```python
from build123d import *

# Parameters (mm, degrees)
BASES_R                     = 6.35
BASE_DEPTH                  = 5.4
TOPBORES_R                  = 1.4
TOP_BORE_DEPTH              = 11.478788098
HORN_START                  = -2.5
HORN_HALF_DEPTH             = 2.5
HORNATTACHS_R               = 0.5
HORN_ATTACH_DEPTH           = 21.913031822
HA_LP_COUNT                 = 4
HA_LP_PITCH                 = 3
HORN_BODIES_COPY_1_SKETCH_R = 0.5
HORN_BODIES_COPY_1_DEPTH    = 21.913031822
HORN_BODIES_COPY_2_SKETCH_R = 0.5
HORN_BODIES_COPY_2_DEPTH    = 21.913031822
HORN_BODIES_COPY_3_SKETCH_R = 0.5
HORN_BODIES_COPY_3_DEPTH    = 21.913031822
TOOTH_DEPTH                 = 3
TOOTH_CP_COUNT              = 26
BOTTOMBORES_R               = 2.6
BOTTOM_BORE_DEPTH           = 3
HOLDINGSHAFTS_R             = 6.35
HOLDINGSHAFTS_R_2           = 4.25
HOLDING_SHAFT_DEPTH         = 2.9
TOPCUTS_R                   = 4.375
TOP_CUT_DEPTH               = 1
TOPPOCKETCYLINDERS_R        = 3.375
TOPPOCKETCYLINDERS_R_2      = 2.875
TOP_POCKET_CYLINDER_DEPTH   = 1.35
CUT_EXTRUDE1_START          = -2.5
CUT_EXTRUDE1_DEPTH          = 2.5


with BuildPart() as part:
    # BaseS → BASE (new body)
    with BuildSketch(Plane(origin=(0, 0, 0), x_dir=(1, 0, 0), z_dir=(0, 1, 0))):
        with Locations(Location((0, 0, 0), (0, 0, 90))):
            Circle(BASES_R)
    extrude(amount=BASE_DEPTH)

    # TopBoreS → TOP BORE (cut, through all)
    with BuildSketch(Plane(origin=(0, 5.4, 0), x_dir=(1, 0, 0), z_dir=(0, 1, 0))):
        with Locations(Location((0, 0, 0), (0, 0, 270))):
            Circle(TOPBORES_R)
    extrude(amount=-TOP_BORE_DEPTH, mode=Mode.SUBTRACT)

    # HornHalfS → HORN HALF (add)
    with BuildSketch(Plane(origin=(0, 5.4, 0), x_dir=(1, 0, 0), z_dir=(0, 1, 0)).offset(HORN_START)):
        with BuildLine():
            Line((-2.609740545, 16.990167671), (-4.891612682, 4.049027706))
            ThreePointArc((-4.891612682, 4.049027706), (0, 6.35), (4.891612682, 4.049027706))
            Line((4.891612682, 4.049027706), (2.609740545, 16.990167671))
            ThreePointArc((2.609740545, 16.990167671), (0, 19.18), (-2.609740545, 16.990167671))
        make_face()
    horn_half = extrude(amount=HORN_HALF_DEPTH)

    # HornAttachS → HORN ATTACH (cut, through all)
    with BuildSketch(Plane(origin=(0, 5.4, 0), x_dir=(1, 0, 0), z_dir=(0, 1, 0))):
        with Locations(Location((0, 16.53, 0), (0, 0, 270))):
            Circle(HORNATTACHS_R)
    horn_attach = extrude(amount=-HORN_ATTACH_DEPTH, mode=Mode.SUBTRACT)

    # HA LP: HORN ATTACH ×4
    with Locations(*[(0, 0, i * HA_LP_PITCH) for i in range(1, HA_LP_COUNT)]):
        add(horn_attach, mode=Mode.SUBTRACT)

    # HORN BODIES: HORN HALF, HORN ATTACH across plane
    add(horn_half.mirror(Plane.XY))
    add(horn_attach.mirror(Plane.XY), mode=Mode.SUBTRACT)

    # HORN BODIES copy 1 sketch → HORN BODIES copy 1 (cut, through all)
    with BuildSketch(Plane(origin=(0, 5.4, -3), x_dir=(1, 0, 0), z_dir=(0, 1, 0))):
        with Locations((0, -16.53)):
            Circle(HORN_BODIES_COPY_1_SKETCH_R)
    extrude(amount=-HORN_BODIES_COPY_1_DEPTH, mode=Mode.SUBTRACT)

    # HORN BODIES copy 2 sketch → HORN BODIES copy 2 (cut, through all)
    with BuildSketch(Plane(origin=(0, 5.4, -6), x_dir=(1, 0, 0), z_dir=(0, 1, 0))):
        with Locations((0, -16.53)):
            Circle(HORN_BODIES_COPY_2_SKETCH_R)
    extrude(amount=-HORN_BODIES_COPY_2_DEPTH, mode=Mode.SUBTRACT)

    # HORN BODIES copy 3 sketch → HORN BODIES copy 3 (cut, through all)
    with BuildSketch(Plane(origin=(0, 5.4, -9), x_dir=(1, 0, 0), z_dir=(0, 1, 0))):
        with Locations((0, -16.53)):
            Circle(HORN_BODIES_COPY_3_SKETCH_R)
    extrude(amount=-HORN_BODIES_COPY_3_DEPTH, mode=Mode.SUBTRACT)

    # ToothS → TOOTH (cut)
    with BuildSketch(Plane.XZ):
        with BuildLine():
            Line((0, -2.9), (0.262912611, -2.586672952))
            ThreePointArc((0.262912611, -2.586672952), (0, -2.6), (-0.262912611, -2.586672952))
            Line((-0.262912611, -2.586672952), (0, -2.9))
        make_face()
    tooth = extrude(amount=-TOOTH_DEPTH, mode=Mode.SUBTRACT)

    # TOOTH CP: TOOTH ×26 about axis
    tooth_cp_axis = Axis((0, 0, 0), (0, 1, 0))
    for i in range(1, TOOTH_CP_COUNT):
        add(tooth.rotate(tooth_cp_axis, i * 360 / TOOTH_CP_COUNT), mode=Mode.SUBTRACT)

    # BottomBoreS → BOTTOM BORE (cut)
    with BuildSketch(Plane(origin=(0, 0, 0), x_dir=(-1, 0, 0), z_dir=(0, -1, 0))):
        Circle(BOTTOMBORES_R)
    extrude(amount=-BOTTOM_BORE_DEPTH, mode=Mode.SUBTRACT)

    # HoldingShaftS → HOLDING SHAFT (cut)
    with BuildSketch(Plane.XZ):
        Circle(HOLDINGSHAFTS_R)
        with Locations(Location((0, 0, 0), (0, 0, 270))):
            Circle(HOLDINGSHAFTS_R_2, mode=Mode.SUBTRACT)
    extrude(amount=-HOLDING_SHAFT_DEPTH, mode=Mode.SUBTRACT)

    # TopCutS → TOP CUT (cut)
    with BuildSketch(Plane(origin=(0, 5.4, 0), x_dir=(1, 0, 0), z_dir=(0, 1, 0))):
        with Locations(Location((0, 0, 0), (0, 0, 270))):
            Circle(TOPCUTS_R)
    extrude(amount=-TOP_CUT_DEPTH, mode=Mode.SUBTRACT)

    # TopPocketCylinderS → TOP POCKET CYLINDER (add)
    with BuildSketch(Plane(origin=(0, 4.4, 0), x_dir=(1, 0, 0), z_dir=(0, 1, 0))):
        with Locations(Location((0, 0, 0), (0, 0, 270))):
            Circle(TOPPOCKETCYLINDERS_R)
        with Locations(Location((0, 0, 0), (0, 0, 270))):
            Circle(TOPPOCKETCYLINDERS_R_2, mode=Mode.SUBTRACT)
    extrude(amount=TOP_POCKET_CYLINDER_DEPTH)

    # Sketch1 → Cut-Extrude1 (cut)
    with BuildSketch(Plane(origin=(0, 5.4, 0), x_dir=(1, 0, 0), z_dir=(0, 1, 0)).offset(CUT_EXTRUDE1_START)):
        with BuildLine():
            Line((4.679848864, -5.25), (2.609740545, -16.990167671))
            ThreePointArc((2.609740545, -16.990167671), (0, -19.18), (-2.609740545, -16.990167671))
            Line((-2.609740545, -16.990167671), (-4.679848864, -5.25))
            Line((-4.679848864, -5.25), (4.679848864, -5.25))
        make_face()
    extrude(amount=CUT_EXTRUDE1_DEPTH, mode=Mode.SUBTRACT)


solid = part.part
```
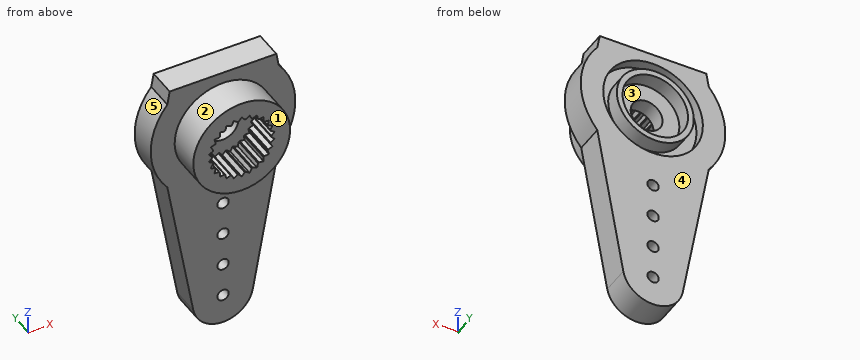
For this review, take the finished solid that the model builds, in its own axes (mm). Face numbers are marked on the shaded views. A direction names the side the tool comes from. Round coordinates to 2 decimals unless told otherwise and drop trailing zeros. Write each loop counter-clockwise with the first axis right and the second up, starting at its lowest first coordinate (ties: lowest second). Pieces come first, ordered by that corner, then holes. Notation, with made-up numbers: (15, -13.5) - (43, -13.5) arc R33 ccw to (43, 19.5) - close; hole circle Ø6 at (84, -33.5). An arc over 180 degrees is marked (long way). Answer as a JSON object with one key per item and string values.
1. To check wall thickness, follow line 1 along X through (y, z) = (4.65, 0) (3 decimals); line 2 along Y through (x, z) = (0, -6.5); line 3 along X through (y, z) = (3.75, -10.53). State the ranges of each line that lie inside material, in increasing order.
Response values:
{"line 1": "x = -6.35 to -4.375, -3.375 to -2.875, 2.875 to 3.375, 4.375 to 6.35", "line 2": "y = 2.9 to 5.4", "line 3": "x = -3.75 to -0.5, 0.5 to 3.75"}
2. Draft analysis for pull direction Z (two halves, no side actions). For the marked faces 3, 4 and 5, state which applies: +Z half, -Z half, draft (parallel to the pull), parting line (faces both ways), or undercut.
Response values:
{"face 3": "undercut", "face 4": "draft", "face 5": "parting line"}
3. We need section C-C on z = -16.75. Give the boundary of the cut face in (x, y), then the cut area to 3 significant figures.
Response values:
{"outline": "(-2.65, 2.9) - (-0.45, 2.9) - (-0.45, 5.4) - (-2.65, 5.4) - close; (0.45, 2.9) - (2.65, 2.9) - (2.65, 5.4) - (0.45, 5.4) - close", "area": "11.0 mm2"}
4. We need section A-A on z = -13.53. Give the boundary of the cut face in (x, y).
Response values:
{"outline": "(-3.22, 2.9) - (-0.5, 2.9) - (-0.5, 5.4) - (-3.22, 5.4) - close; (0.5, 2.9) - (3.22, 2.9) - (3.22, 5.4) - (0.5, 5.4) - close"}
5. For pin 1 Ø5 at (x, z) = (0, 0) entering from +Y; pin 2 Ø3 at (x, z) = (0, 0) entering from -Y; pin 3 Ø3 at (y, z) = (1, -4.5) entering from +X; pin 4 Ø1.5 at (x, z) = (1, -2) entering from -Y, all flat-tipped, find the tip position at first contact; note any pin that passes through.
Response values:
{"pin 1": "stops at y = 4.4", "pin 2": "stops at y = 3", "pin 3": "stops at x = 3.01", "pin 4": "stops at y = 0"}
6. Tool access review of the marked faces 1 and 2: name each direction out of +Z, -Z, +X, -X, +Y, -Y from which nothing blocks a thin tool from reaching the whole face with its end or side.
Response values:
{"face 1": "+Z, -Z, +X, -X, -Y", "face 2": "-Y"}
7. We need section B-B on y = 3.7. Give the boundary of the cut face in (x, z).
Response values:
{"outline": "(-4.89, -4.05) - (-2.61, -16.99) arc R2.65 ccw to (2.61, -16.99) - (4.89, -4.05) arc R6.35 ccw to (4.89, 4.05) - (4.68, 5.25) - (-4.68, 5.25) - (-4.89, 4.05) arc R6.35 ccw to start; hole circle Ø2.8 at (0, 0); hole circle Ø1 at (0, -16.53); hole circle Ø1 at (0, -13.53); hole circle Ø1 at (0, -10.53); hole circle Ø1 at (0, -7.53)"}
